from build123d import *

# Parameters (mm, degrees)
BOSS_EXTRUDE2_DEPTH = 4
CUT_EXTRUDE1_DEPTH  = 3.75
CUT_EXTRUDE2_START  = 7.5
CUT_EXTRUDE2_DEPTH  = 7.5
SKETCH2_R           = 0.205
CUT_EXTRUDE3_DEPTH  = 7.5


with BuildPart() as part:
    # Sketch1 → Boss-Extrude2 (new, symmetric)
    with BuildSketch(Plane(origin=(0, 0, 0), x_dir=(1, 0, 0), z_dir=(0, 1, 0))):
        with BuildLine():
            Line((-1.5, 0), (-4.88, 0))
            ThreePointArc((-4.88, 0), (0, -4.88), (4.88, 0))
            Line((4.88, 0), (1.5, 0))
            ThreePointArc((1.5, 0), (0, -1.5), (-1.5, 0))
        make_face()
        with BuildLine():
            ThreePointArc((3.31662479, -5), (0, -6), (-3.31662479, -5))
            Line((-3.31662479, -5), (-7, -5))
            Line((-7, -5), (-7, -6.5))
            Line((-7, -6.5), (7, -6.5))
            Line((7, -6.5), (7, -5))
            Line((7, -5), (3.31662479, -5))
        make_face()
        with BuildLine():
            Line((-4.88, 0), (-5.75, 0))
            ThreePointArc((-5.75, 0), (0, -5.75), (5.75, 0))
            Line((5.75, 0), (4.88, 0))
            ThreePointArc((4.88, 0), (0, -4.88), (-4.88, 0))
        make_face()
        with BuildLine():
            Line((-5.75, 0), (-7.5, 0))
            Line((-7.5, 0), (-7.5, -0.41))
            Line((-7.5, -0.41), (-5.985975276, -0.41))
            ThreePointArc((-5.985975276, -0.41), (-5.186676874, -3.016352599), (-3.31662479, -5))
            ThreePointArc((-3.31662479, -5), (0, -6), (3.31662479, -5))
            ThreePointArc((3.31662479, -5), (5.186676874, -3.016352599), (5.985975276, -0.41))
            Line((5.985975276, -0.41), (7.5, -0.41))
            Line((7.5, -0.41), (7.5, 0))
            Line((7.5, 0), (5.75, 0))
            ThreePointArc((5.75, 0), (0, -5.75), (-5.75, 0))
        make_face()
    extrude(amount=BOSS_EXTRUDE2_DEPTH, both=True)

    # Sketch1_3 → Cut-Extrude1 (cut, symmetric)
    with BuildSketch(Plane(origin=(0, 0, 0), x_dir=(1, 0, 0), z_dir=(0, 1, 0))):
        with BuildLine():
            Line((-1.5, 0), (-4.88, 0))
            ThreePointArc((-4.88, 0), (0, -4.88), (4.88, 0))
            Line((4.88, 0), (1.5, 0))
            ThreePointArc((1.5, 0), (0, -1.5), (-1.5, 0))
        make_face()
        with BuildLine():
            Line((-4.88, 0), (-5.75, 0))
            ThreePointArc((-5.75, 0), (0, -5.75), (5.75, 0))
            Line((5.75, 0), (4.88, 0))
            ThreePointArc((4.88, 0), (0, -4.88), (-4.88, 0))
        make_face()
    extrude(amount=CUT_EXTRUDE1_DEPTH, both=True, mode=Mode.SUBTRACT)

    # Sketch1_4 → Cut-Extrude2 (cut)
    with BuildSketch(Plane(origin=(0, 0, 0), x_dir=(1, 0, 0), z_dir=(0, 1, 0)).offset(CUT_EXTRUDE2_START)):
        with BuildLine():
            Line((-1.5, 0), (-4.88, 0))
            ThreePointArc((-4.88, 0), (0, -4.88), (4.88, 0))
            Line((4.88, 0), (1.5, 0))
            ThreePointArc((1.5, 0), (0, -1.5), (-1.5, 0))
        make_face()
    extrude(amount=-CUT_EXTRUDE2_DEPTH, mode=Mode.SUBTRACT)

    # Sketch2 → Cut-Extrude3 (cut)
    with BuildSketch(Plane.XY.offset(0.41)):
        with Locations((-6.75, 3)):
            Circle(SKETCH2_R)
        with Locations((-6.75, 1)):
            Circle(SKETCH2_R)
        with Locations(Location((-6.75, -1, 0), (0, 0, 180))):
            Circle(SKETCH2_R)
        with Locations(Location((-6.75, -3, 0), (0, 0, 180))):
            Circle(SKETCH2_R)
        with Locations((6.75, -3)):
            Circle(SKETCH2_R)
        with Locations((6.75, -1)):
            Circle(SKETCH2_R)
        with Locations(Location((6.75, 1, 0), (0, 0, 180))):
            Circle(SKETCH2_R)
        with Locations(Location((6.75, 3, 0), (0, 0, 180))):
            Circle(SKETCH2_R)
    extrude(amount=-CUT_EXTRUDE3_DEPTH, mode=Mode.SUBTRACT)


solid = part.part
The model under review builds one solid part; all positions refer to its coordinate system, in mm. A direction names the side the tool comes from. Give positions to 0.01 mm unless a question says otherwise; leave off trailing zeros. Loops run counter-clockwise (first coordinate to the right, second up) from the corner with the lowest first, then second, coordinate; pieces in that order, holes last. Notation, with made-up numbers: (57.25, 36.25) -> (74.25, 36.25) arc R19 ccw to (74.25, 53.25) -> close; hole circle Ø9 at (85, -28). An arc over 180 degrees is marked (long way). Answer as a JSON object with one key per item and string values. Group by question number.
Q1. Take a section at D-D (y = -0.5). Write out the cut boundary in (x, z), plus the area to 3 significant figures.
Q2. Tool access review of faces 4 (the flat face through (-7, 0, 0.41)), 5 (the flat face through (5, 0, 5)), 6 (the cylindrical face through (-0.13, 0.05, 5.75)): name each direction out of +Z, -Z, +X, -X, +Y, -Y from which nothing blocks a thin tool from reaching the whole face with its end or side.
Q3. Take a section at B-B (y = 1). Write out the cut boundary in (x, z) (3 decimals), plus the area to 3 significant figures.
Q4. Take a section at A-A (x = 6.75). Write out the cut boundary in (y, z) (3 decimals), plus the area to 3 significant figures.
Q5. Insertion check: pin 1 (4 mm diameter, centred on x = 5.5, y = -1.5, fed in from -Z); pin 2 (3 mm diameter, centred on x = -2, z = 2.5, fed in from +Y); pin 3 (0.8 mm diameter, centred on y = 0, z = 6, fed in from +X); pin 4 (1.1 mm diameter, centred on x = -4.5, y = 0.5, fed in from -Z). Each pin has a flat end and moves straight along its axis. Give the tip position at first contact, or say it passes through.
Q6. Wall thickness on line 1 along Y through (x, z) = (-6.75, 0.2) (3 decimals); line 2 along Y through (x, z) = (-3.75, 3.75); line 3 along Z through (x, y) = (6.75, 1.5): over which ranges is each line inside the solid? List them lowest first.
Q7. Take a section at C-C (z = 5.5). Write out the cut boundary in (x, y), plus the area to 3 significant figures.
Q8. Draft analysis for pull direction X (two halves, no side actions). For faces 1 (the flat face through (-6, 0, 0)), 2 (the flat face through (0, -3.75, 3)), 3 (the flat face through (7, 0, 6)), state which applies: pulls with the +X half, pulls with the -X half, needs draft (parallel to the pull), parting line crosses it, or undercut.
Answer below:
{
 "1": {"outline": "(-7.5, 0) -> (-5.75, 0) arc R5.75 cw to (5.75, 0) -> (7.5, 0) -> (7.5, 0.41) -> (5.99, 0.41) arc R6 ccw to (3.32, 5) -> (7, 5) -> (7, 6.5) -> (-7, 6.5) -> (-7, 5) -> (-3.32, 5) arc R6 ccw to (-5.99, 0.41) -> (-7.5, 0.41) -> close", "area": "22.3 mm2"},
 "2": {"face 4": "-X, +Y, -Y", "face 5": "+X, +Y, -Y", "face 6": "-Z"},
 "3": {"outline": "(-7.5, 0) -> (-6.955, 0) -> (-6.955, 0.41) -> (-7.5, 0.41) -> close; (-7, 5) -> (-3.317, 5) arc R6 ccw to (-5.986, 0.41) -> (-6.545, 0.41) -> (-6.545, 0) -> (-5.75, 0) arc R5.75 cw to (5.75, 0) -> (6.545, 0) -> (6.545, 0.41) -> (5.986, 0.41) arc R6 ccw to (3.317, 5) -> (7, 5) -> (7, 6.5) -> (-7, 6.5) -> close; (6.955, 0) -> (7.5, 0) -> (7.5, 0.41) -> (6.955, 0.41) -> close", "area": "22.0 mm2"},
 "4": {"outline": "(-4, 0) -> (-3.205, 0) -> (-3.205, 0.41) -> (-4, 0.41) -> close; (-4, 5) -> (4, 5) -> (4, 6.5) -> (-4, 6.5) -> close; (-2.795, 0) -> (-1.205, 0) -> (-1.205, 0.41) -> (-2.795, 0.41) -> close; (-0.795, 0) -> (0.795, 0) -> (0.795, 0.41) -> (-0.795, 0.41) -> close; (1.205, 0) -> (2.795, 0) -> (2.795, 0.41) -> (1.205, 0.41) -> close; (3.205, 0) -> (4, 0) -> (4, 0.41) -> (3.205, 0.41) -> close", "area": "14.6 mm2"},
 "5": {"pin 1": "stops at z = 0", "pin 2": "stops at y = -3.75", "pin 3": "stops at x = 7", "pin 4": "stops at z = 2.75"},
 "6": {"line 1": "y = -4 to -3.205, -2.795 to -1.205, -0.795 to 0.795, 1.205 to 2.795, 3.205 to 4", "line 2": "y = -4 to -3.75, 3.75 to 4", "line 3": "z = 0 to 0.41, 5 to 6.5"},
 "7": {"outline": "(-7, -4) -> (7, -4) -> (7, 4) -> (-7, 4) -> close; hole (-1.68, -3.75) -> (1.68, -3.75) -> (1.68, 3.75) -> (-1.68, 3.75) -> close", "area": "86.8 mm2"},
 "8": {"face 1": "needs draft", "face 2": "undercut", "face 3": "pulls with the +X half"}
}
